Work out the finished part from the listing and answer in its coordinate system (mm). A direction names the side the tool comes from. Round coordinates to 2 decimals unless told otherwise and drop trailing zeros. Loops run counter-clockwise (first coordinate to the right, second up) from the corner with the lowest first, then second, coordinate; pieces in that order, holes last.
```python
from build123d import *

# Parameters (mm, degrees)
BOSS_EXTRUDE1_DEPTH = 7
BOSS_EXTRUDE2_DEPTH = 6
BOSS_EXTRUDE3_DEPTH = 7
SKETCH4_R           = 0.3
BOSS_EXTRUDE4_DEPTH = 1.75


with BuildPart() as part:
    # Sketch1 → Boss-Extrude1 (new, symmetric)
    with BuildSketch(Plane.XY):
        with BuildLine():
            Line((9.176470588, 3.852941176), (9.176470588, 8.382352941))
            Line((9.176470588, 8.382352941), (3.176470588, 8.382352941))
            Line((3.176470588, 8.382352941), (3.176470588, 6.352941176))
            Line((3.176470588, 6.352941176), (-11.058823529, 6.352941176))
            ThreePointArc((-11.058823529, 6.352941176), (-12.473037092, 5.767154739), (-13.058823529, 4.352941176))
            Line((-13.058823529, 4.352941176), (-13.058823529, 3.852941176))
            Line((-13.058823529, 3.852941176), (9.176470588, 3.852941176))
        make_face()
    extrude(amount=BOSS_EXTRUDE1_DEPTH, both=True)

    # Sketch2 → Boss-Extrude2 (add, symmetric)
    with BuildSketch(Plane.XY):
        with BuildLine():
            Line((-13.058823529, 3.852941176), (-13.058823529, 2.660454677))
            ThreePointArc((-13.058823529, 2.660454677), (-12.542636873, 1.319448352), (-11.260525567, 0.670651599))
            Line((-11.260525567, 0.670651599), (3.072810241, -0.782287673))
            Line((3.072810241, -0.782287673), (3.072810241, 0.357643739))
            Line((3.072810241, 0.357643739), (-10.868321542, 1.982265031))
            ThreePointArc((-10.868321542, 1.982265031), (-11.499481128, 2.310618881), (-11.752570466, 2.975543285))
            Line((-11.752570466, 2.975543285), (-11.752570466, 3.852941176))
            Line((-11.752570466, 3.852941176), (-13.058823529, 3.852941176))
        make_face()
    extrude(amount=BOSS_EXTRUDE2_DEPTH, both=True)

    # Sketch3 → Boss-Extrude3 (add, symmetric)
    with BuildSketch(Plane.XY):
        with BuildLine():
            Line((2.883131421, 0.205607724), (3.042051607, -0.684345316))
            ThreePointArc((3.042051607, -0.684345316), (3.191971306, -0.960915025), (3.477393899, -1.0932051))
            Line((3.477393899, -1.0932051), (17.397932492, -2.686911621))
            ThreePointArc((17.397932492, -2.686911621), (17.787643477, -2.563275633), (17.954803987, -2.190156518))
            Line((17.954803987, -2.190156518), (17.954803987, -1.828059238))
            ThreePointArc((17.954803987, -1.828059238), (17.833783341, -1.50190797), (17.529305388, -1.333640851))
            Line((17.529305388, -1.333640851), (3.449846609, 0.78792143))
            ThreePointArc((3.449846609, 0.78792143), (3.017025208, 0.642224676), (2.883131421, 0.205607724))
        make_face()
    extrude(amount=BOSS_EXTRUDE3_DEPTH, both=True)

    # Sketch4 → Boss-Extrude4 (add, symmetric)
    with BuildSketch(Plane.XY):
        with BuildLine():
            Line((15.880495921, 8.784024701), (31.318309496, 14.894554405))
            ThreePointArc((31.318309496, 14.894554405), (34.7916946, 15.766688386), (32.722657859, 12.843657643))
            Line((32.722657859, 12.843657643), (15.583027287, 4.472426378))
            add(Edge.make_bspline(
                [(9.176470588, 3.852941176), (12.411471434, 3.711455216), (15.583027287, 4.472426378)],
                knots=[0, 0, 0, 1, 1, 1], degree=2))
            Line((9.176470588, 3.852941176), (9.176470588, 8.382352941))
            add(Edge.make_bspline(
                [(9.176470588, 8.382352941), (12.540784879, 8.295907329), (15.880495921, 8.784024701)],
                knots=[0, 0, 0, 1, 1, 1], degree=2))
        make_face()
        with Locations((33.216362624, 14.687982269)):
            Circle(SKETCH4_R, mode=Mode.SUBTRACT)
    extrude(amount=BOSS_EXTRUDE4_DEPTH, both=True)


solid = part.part
```
1. Which of the six approach directions +Z, -Z, +X, -X, +Y, -Y give full straight-line access (tool end or side, diameter ignored) to faces 1 (the face through (3.176, 7, 0)), 2 (the face through (9.176, 6, 4)), 3 (the face through (-6, 1, -6))?
Answer key:
face 1: +Z, -Z, -X, +Y
face 2: +Z, +X, +Y
face 3: -Z, -X, -Y
2. Given pin 1 (5 mm diameter, centred on x = 9.5, z = 4, fed in from -Y); pin 2 (1.4 mm diameter, centred on y = 7, z = -3.5, fed in from +X); pin 3 (7 mm diameter, centred on x = -6, z = 1, fed in from -Y), each flat-ended and moving along its own axis, determine where each tip first touches the part or whether it passes through.
Answer key:
pin 1: stops at y = -2.07
pin 2: stops at x = 9.18
pin 3: stops at y = -0.22
3. Find section B-B (z = 4.5). Write down the section's boundary in (x, y).
Answer key:
outline: (-13.06, 2.66) arc R2 ccw to (-11.26, 0.67) - (3.07, -0.78) arc R0.5 ccw to (3.48, -1.09) - (17.4, -2.69) arc R0.5 ccw to (17.95, -2.19) - (17.95, -1.83) arc R0.5 ccw to (17.53, -1.33) - (3.45, 0.79) arc R0.5 ccw to (2.88, 0.38) - (-10.87, 1.98) arc R1 cw to (-11.75, 2.98) - (-11.75, 3.85) - (9.18, 3.85) - (9.18, 8.38) - (3.18, 8.38) - (3.18, 6.35) - (-11.06, 6.35) arc R2 ccw to (-13.06, 4.35) - close
4. Find section A-A (x = -8). Write down the section's boundary in (y, z).
Answer key:
outline: (0.34, -6) - (1.65, -6) - (1.65, 6) - (0.34, 6) - close; (3.85, -7) - (6.35, -7) - (6.35, 7) - (3.85, 7) - close
5. Find section D-D (y = 11). Write down the section's boundary in (x, z).
Answer key:
outline: (21.48, -1.75) - (28.95, -1.75) - (28.95, 1.75) - (21.48, 1.75) - close
6. Consider probe 1 along Y at (x, z) = (-3, 4.25); probe 2 along Y at (x, z) = (6, -5.75); probe 3 along X at (y, z) = (3.25, 2). Determine where each line is inside the solid, lowest interval first.
Answer key:
probe 1: y = -0.17 to 1.07, 3.85 to 6.35
probe 2: y = -1.38 to 0.4, 3.85 to 8.38
probe 3: x = -13.06 to -11.75
7. Find section C-C (x = 5). Write down the section's boundary in (y, z).
Answer key:
outline: (-1.27, -7) - (0.55, -7) - (0.55, 7) - (-1.27, 7) - close; (3.85, -7) - (8.38, -7) - (8.38, 7) - (3.85, 7) - close
8. Determine the mould class of faces 4 (the face through (-4, 6.353, 0)), 5 (the face through (21, 10, -1.75)), 6 (the face through (-11.753, 3.4, 0.1)), 7 (the face through (-3.9, 1.17, 0.08)) for opening direction Y: +Y half, -Y half, draft (parallel to the pull), parting line (faces both ways), or undercut.
Answer key:
face 4: +Y half
face 5: draft
face 6: undercut
face 7: undercut
